CAD build for the part. Positions are in the model's coordinates, mm. Round coordinates to 2 decimals unless told otherwise and drop trailing zeros. Write each loop counter-clockwise with the first axis right and the second up, starting at its lowest first coordinate (ties: lowest second). Pieces come first, ordered by that corner, then holes. Notation, with made-up numbers: (-25, -15.5) - (-21, -15.5) arc R33 cw to (-21, 21.5) - close; hole circle Ø8 at (81.25, -20.5). An arc over 180 degrees is marked (long way). Put each result on its own line as item: value. Start each with the question number.
Item 1: Pin check, flat tips, straight feed: pin 1 Ø2.5 at (x, y) = (4.76, 4.76) entering from +Z; pin 2 Ø2 at (x, y) = (123, 5) entering from -Z (3 decimals). Stop position of each tip, or through.
Item 2: Cut at A-A (x = 54). Give the cut face in (y, z) (3 decimals).
Item 3: Drill centre lines: line 1 (X direction, y = 5, z = -64) (3 decimals); line 2 (X direction, y = 8, z = -64.5) (3 decimals); line 3 (X direction, y = 3, z = -68.5) (3 decimals). Where is each one in solid material? Low to high. Write a range as from..to.
Item 4: Cut at B-B (z = -42). Give the cut face in (x, y) (3 decimals), and give its area (3 significant figures).
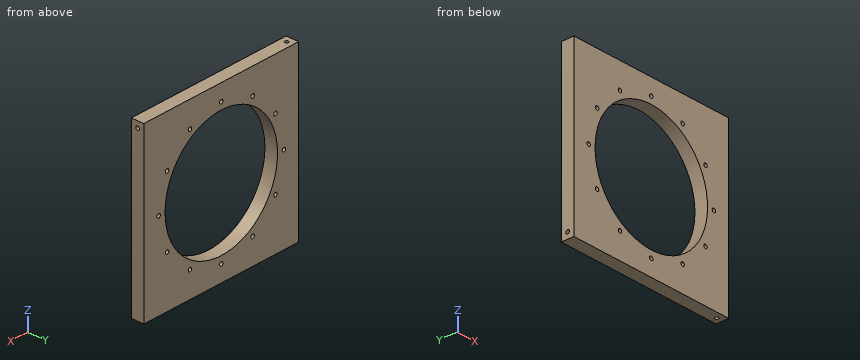
```python
from build123d import *

# Parameters (mm, degrees)
SKETCH1_W           = 127.635
SKETCH1_H           = 127.635
BOSS_EXTRUDE1_DEPTH = 9.525
SKETCH5_R           = 46.355
CUT_EXTRUDE1_DEPTH  = 9.525
SKETCH11_R          = 1.4351
CUT_EXTRUDE3_DEPTH  = 10.525
CIRPATTERN1_COUNT   = 12
SKETCH6_R           = 1.35255
F_6_32_HOLE1_DEPTH  = 12.7
SKETCH7_R           = 1.35255
F_6_32_HOLE2_DEPTH  = 12.7
SKETCH8_R           = 1.35255
F_6_32_HOLE3_DEPTH  = 12.7
SKETCH9_R           = 1.35255
F_6_32_HOLE4_DEPTH  = 12.7


with BuildPart() as part:
    # Sketch1 → Boss-Extrude1 (new body)
    with BuildSketch(Plane(origin=(0, 0, 0), x_dir=(1, 0, 0), z_dir=(0, 1, 0))):
        with Locations((63.8175, 63.8175)):
            Rectangle(SKETCH1_W, SKETCH1_H)
    extrude(amount=BOSS_EXTRUDE1_DEPTH)

    # Sketch5 → Cut-Extrude1 (cut)
    with BuildSketch(Plane(origin=(0, 9.525, 0), x_dir=(1, 0, 0), z_dir=(0, 1, 0))):
        with Locations((63.8175, 63.8175)):
            Circle(SKETCH5_R)
    extrude(amount=-CUT_EXTRUDE1_DEPTH, mode=Mode.SUBTRACT)

    # Sketch11 → Cut-Extrude3 (cut, through all)
    with BuildSketch(Plane(origin=(0, 9.525, 0), x_dir=(1, 0, 0), z_dir=(0, 1, 0))):
        with Locations((63.8175, 115.443)):
            Circle(SKETCH11_R)
    cut_extrude3 = extrude(amount=-CUT_EXTRUDE3_DEPTH, mode=Mode.SUBTRACT)

    # CirPattern1: Cut-Extrude3 ×12 about axis
    cirpattern1_axis = Axis((63.8175, 0, -63.8175), (0, 1, 0))
    for i in range(1, CIRPATTERN1_COUNT):
        add(cut_extrude3.rotate(cirpattern1_axis, i * 360 / CIRPATTERN1_COUNT), mode=Mode.SUBTRACT)

    # Sketch6 → 6-32 hole1 (cut)
    with BuildSketch(Plane(origin=(127.635, 0, 0), x_dir=(0, 0, -1), z_dir=(1, 0, 0))):
        with Locations((4.7625, 4.7625)):
            Circle(SKETCH6_R)
    extrude(amount=-F_6_32_HOLE1_DEPTH, mode=Mode.SUBTRACT)

    # Sketch7 → 6-32 hole2 (cut)
    with BuildSketch(Plane(origin=(0, 0, -127.635), x_dir=(-1, 0, 0), z_dir=(0, 0, -1))):
        with Locations((-122.8725, 4.7625)):
            Circle(SKETCH7_R)
    extrude(amount=-F_6_32_HOLE2_DEPTH, mode=Mode.SUBTRACT)

    # Sketch8 → 6-32 hole3 (cut)
    with BuildSketch(Plane.ZY):
        with Locations((-122.8725, 4.7625)):
            Circle(SKETCH8_R)
    extrude(amount=-F_6_32_HOLE3_DEPTH, mode=Mode.SUBTRACT)

    # Sketch9 → 6-32 hole4 (cut)
    with BuildSketch(Plane.XY):
        with Locations((4.7625, 4.7625)):
            Circle(SKETCH9_R)
    extrude(amount=-F_6_32_HOLE4_DEPTH, mode=Mode.SUBTRACT)


solid = part.part
```
Output values:
1. pin 1: z = -12.7
1. pin 2: z = -114.935
2. outline: (0, -127.635) - (9.525, -127.635) - (9.525, -109.121) - (0, -109.121) - close; (0, -18.514) - (9.525, -18.514) - (9.525, 0) - (0, 0) - close
3. line 1: 0..10.769, 13.615..17.463, 110.172..114.02, 116.866..127.635
3. line 2: 0..10.93, 13.454..17.468, 110.167..114.181, 116.705..127.635
3. line 3: 0..17.7, 109.935..127.635
4. outline: (0, 0) - (22.918, 0) - (22.918, 9.525) - (0, 9.525) - close; (104.717, 0) - (127.635, 0) - (127.635, 9.525) - (104.717, 9.525) - close
4. area: 437 mm2
